Autodesk Inventor part; units mm, degrees
ref_plane "YZ Plane" through (0, 0, 0) normal (1, 0, 0) x (0, 1, 0)
ref_plane "XZ Plane" through (0, 0, 0) normal (0, 1, 0) x (-1, 0, 0)
ref_plane "XY Plane" through (0, 0, 0) normal (0, 0, 1) x (1, 0, 0)
sketch "Sketch8" plane through (0, 0, 3) normal (0, 0, 1) x (1, 0, 0)
  line L0 (-83.75, -130) -> (-83.75, 220)
  line L1 (-83.75, 220) -> (-89.75, 220)
  line L2 (-89.75, 220) -> (-89.75, -130)
  line L3 (-89.75, -130) -> (-83.75, -130)
  line L4 (-83.75, -130) -> (-83.75, 220)
  line L5 (-86.75, -130) -> (-86.75, 0)
  line L6 (-86.75, 0) -> (-83.75, 0)
  point P0 (0, 0)
  dimension "d35" = 6
sketch "Sketch1" plane through (0, 0, 0) normal (0, 0, 1) x (1, 0, 0)
  line L0 (-83.75, -220) -> (83.75, -220)
  line L1 (83.75, -220) -> (83.75, 220)
  line L2 (83.75, 220) -> (-83.75, 220)
  line L3 (-83.75, 220) -> (-83.75, -220)
  line L4 (-83.75, -220) -> (83.75, 220) construction
  line L5 (83.75, -220) -> (-83.75, 220) construction
  point P0 (0, 0)
  dimension "d0" = 440
  dimension "d1" = 167.5
extrude "Plate1" add sketch "Sketch1" along normal blind 3
sketch "Sketch3" plane through (0, 0, 3) normal (0, 0, 1) x (1, 0, 0)
  line L0 (-83.75, -220) -> (83.75, -220)
  line L1 (-83.75, -220) -> (-23.75, -220)
  line L2 (-23.75, -220) -> (-23.75, -130)
  line L3 (-23.75, -130) -> (-83.75, -130)
  line L4 (-83.75, -130) -> (-83.75, -220)
  point P0 (0, 0)
  dimension "d7" = 60
  dimension "d8" = 90
extrude "Cut2" cut sketch "Sketch3" against normal blind 3
sketch "Sketch4" plane through (0, 0, 3) normal (0, 0, 1) x (1, 0, 0)
  line L0 (-83.75, 220) -> (-83.75, -130)
  line L1 (-28.75, -88) -> (-3.75, -88)
  line L2 (-3.75, -88) -> (-3.75, -118)
  line L3 (-3.75, -118) -> (-83.75, -118)
  line L4 (-83.75, -118) -> (-83.75, -93)
  line L5 (-83.75, -130) -> (-23.75, -130)
  line L6 (-28.75, -88) -> (-28.75, -118)
  point P0 (0, 0)
  dimension "d11" = 12
  dimension "d12" = 30
  dimension "d13" = 25
  dimension "d16" = 55
extrude "Cut3" cut sketch "Sketch4" against normal blind 3
sketch "Sketch5" plane through (0, 0, 3) normal (0, 0, 1) x (1, 0, 0)
  line L0 (-33.75, 195) -> (-28.75, 195)
  line L1 (-28.75, 195) -> (-28.75, -130)
  line L2 (-28.75, -130) -> (-33.75, -130)
  line L3 (-33.75, -130) -> (-33.75, 195)
  line L4 (-83.75, 220) -> (83.75, 220)
  line L5 (-83.75, -130) -> (-23.75, -130)
  line L6 (-83.75, -130) -> (-83.75, 220)
  point P0 (0, 0)
  point P1 (-31.25, -130)
  dimension "d17" = 25
  dimension "d18" = 5
  dimension "d19" = 50
extrude "Cut4" cut sketch "Sketch5" against normal blind 3
fillet "Corner Round1" radius 5 1 edges at (83.75, 220, 1.5)
sketch "Sketch6" plane through (0, 0, 3) normal (0, 0, 1) x (1, 0, 0)
  line L0 (83.75, 215) -> (83.75, -220)
  line L1 (83.75, 217) -> (33.75, 217)
  line L2 (33.75, 217) -> (33.75, 214)
  line L3 (33.75, 214) -> (83.75, 214)
  line L4 (83.75, 214) -> (83.75, 217)
  line L5 (-83.75, 220) -> (78.75, 220)
  point P0 (0, 0)
  point P1 (-78.75, 220)
  dimension "d24" = 50
  dimension "d25" = 3
  dimension "d26" = 3
extrude "Cut5" cut sketch "Sketch6" against normal blind 3
sketch "Sketch7" plane through (0, 0, 3) normal (0, 0, 1) x (1, 0, 0)
  line L0 (76.75, 122) -> (79.75, 122)
  line L1 (79.75, 122) -> (79.75, -128)
  line L2 (79.75, -128) -> (76.75, -128)
  line L3 (76.75, -128) -> (76.75, 122)
  line L4 (83.75, 214) -> (83.75, -220)
  line L5 (83.75, -220) -> (-23.75, -220)
  point P0 (0, 0)
  dimension "d29" = 3
  dimension "d30" = 4
  dimension "d31" = 92
  dimension "d32" = 250
extrude "Cut6" cut sketch "Sketch7" against normal blind 3
sheet face with bend "Face2" sketch "Sketch8" thickness 3 toward (0, 0, -1) bend radius 3 contours L6 L5 L3 L2 L1 L0
bend "Bend1"
equation "\"d9\" = Thickness"
equation "\"d14\" = Thickness"
equation "\"d20\" = Thickness"
equation "\"d27\" = Thickness"
equation "\"d33\" = Thickness"
equation "\"d2\" = Thickness"
equation "\"d36\" = BendRadius"
equation "\"d37\" = BendReliefWidth"
equation "\"d39\" = MinimumRemnant"
equation "\"d38\" = BendReliefDepth"
equation "\"d40\" = TransitionRadius"
equation "\"BendRadius\" = Thickness"
equation "\"BendReliefWidth\" = Thickness"
equation "\"BendReliefDepth\" = 0.5 * Thickness"
equation "\"CornerReliefSize\" = 4 * Thickness"
equation "\"MinimumRemnant\" = 2 * Thickness"
equation "\"TransitionRadius\" = BendRadius"
equation "\"JacobiRadiusSize\" = BendRadius"
equation "\"GapSize\" = Thickness"
properties part number "Finishing Sheets .1  ( Right )"
For this review, take the finished solid that the model builds, in its own axes (mm). Give positions to 0.01 mm unless a question says otherwise; leave off trailing zeros. Order: outer loops, then holes, each group sorted by start corner. A loop starts at its lowest first (then second) coordinate and runs counter-clockwise, first axis right, second up. Notation, with made-up numbers: M -8,61.25 L 28,61.25 A22 ccw 28,79.25 Z; hole C 39,48.25 d2. An arc over 180 degrees is marked long. Answer in a Markdown table with one row per item. Add a question column.
(1) Wall thickness on probe 1 along X at (y, z) = (58.5, 2.3); probe 2 along X at (y, z) = (149.5, 0.8); probe 3 along Y at (x, z) = (-15.5, 1.4): over which ranges is each line inside the solid? List them lowest first. Write a range as [from, to].
(2) Consider section C-C on z = 1.35. State the section outline as (x, y) points, and give its area (3 significant figures).
(3) Consider section A-A on y = 115. State the section outline as (x, z) points, and give its area (4 significant figures).
(4) Consider section D-D on x = -8.5. State the section outline as (y, z) points.
(5) Consider section B-B on y = -76. State the section outline as (x, z) points, and give its area (4 significant figures).
(6) For pin 1 (0.9 mm diameter, centred on x = -61, z = 2, fed in from -Y), flat-tipped, find the tip position at first contact; note if it passes through.
Evaluation:
| question | item | result |
|---|---|---|
| 1 | probe 1 | x = [-89.75, -33.75], [-28.75, 76.75], [79.75, 83.75] |
| 1 | probe 2 | x = [-89.75, -33.75], [-28.75, 83.75] |
| 1 | probe 3 | y = [-220, -118], [-88, 220] |
| 2 | outline | M -89.75,-130 L -86.75,-130 L -86.75,0 L -83.75,0 L -83.75,-130 L -33.75,-130 L -33.75,195 L -28.75,195 L -28.75,-88 L -3.75,-88 L -3.75,-118 L -28.75,-118 L -28.75,-130 L -23.75,-130 L -23.75,-220 L 83.75,-220 L 83.75,214 L 33.75,214 L 33.75,217 L 83.33,217 A5 ccw 78.75,220 L -89.75,220 Z; hole M 76.75,-128 L 79.75,-128 L 79.75,122 L 76.75,122 Z |
| 2 | area | 66,700 mm^2 |
| 3 | outline | M -89.75,0 L -33.75,0 L -33.75,3 L -89.75,3 Z; M -28.75,0 L 76.75,0 L 76.75,3 L -28.75,3 Z; M 79.75,0 L 83.75,0 L 83.75,3 L 79.75,3 Z |
| 3 | area | 496.5 mm^2 |
| 4 | outline | M -220,0 L -118,0 L -118,3 L -220,3 Z; M -88,0 L 220,0 L 220,3 L -88,3 Z |
| 5 | outline | M -89.75,0 L -86.75,0 L -86.75,3 L -89.75,3 Z; M -83.75,0 L -33.75,0 L -33.75,3 L -83.75,3 Z; M -28.75,0 L 76.75,0 L 76.75,3 L -28.75,3 Z; M 79.75,0 L 83.75,0 L 83.75,3 L 79.75,3 Z |
| 5 | area | 487.5 mm^2 |
| 6 | pin 1 | stops at y = -130 |
